from build123d import *

# Parameters (mm, degrees)
SKETCH1_W           = 12
SKETCH1_H           = 18.25
SKETCH2_R           = 3.7145
CUT_EXTRUDE1_DEPTH  = 8.5725
SKETCH3_W           = 73.152
SKETCH3_H           = 124
BOSS_EXTRUDE1_DEPTH = 8
FILLET1_R           = 4
SKETCH6_R           = 13.15
CUT_EXTRUDE2_DEPTH  = 12
SKETCH12_R          = 4.075
CUT_EXTRUDE6_DEPTH  = 2.56
SKETCH12_6_R        = 2.5
CUT_EXTRUDE7_DEPTH  = 8
FILLET2_R           = 0.5
SKETCH13_W          = 73.152
SKETCH13_H          = 13.5
SKETCH13_H_2        = 10
BOSS_EXTRUDE3_DEPTH = 15
FILLET3_R           = 2
SKETCH14_R          = 3.71375
CUT_EXTRUDE8_DEPTH  = 9.5


with BuildPart() as part:
    # Sketch1 → Revolve1 (revolve)
    with BuildSketch(Plane.XY):
        with Locations((14.255, 9.125)):
            Rectangle(SKETCH1_W, SKETCH1_H)
    revolve(axis=Axis((8.255, 0, 0), (1, 0, 0)))

    # Sketch2 → Cut-Extrude1 (cut)
    with BuildSketch(Plane.ZY.offset(-8.255)):
        Circle(SKETCH2_R)
    extrude(amount=-CUT_EXTRUDE1_DEPTH, mode=Mode.SUBTRACT)

    # Sketch6 → Cut-Extrude2 (cut)
    with BuildSketch(Plane.ZY.offset(-8.255)):
        Circle(SKETCH6_R)
    extrude(amount=-CUT_EXTRUDE2_DEPTH, mode=Mode.SUBTRACT)


with BuildPart() as body_2:
    # Sketch3 → Boss-Extrude1 (new body)
    with BuildSketch(Plane(origin=(20.255, 0, 0), x_dir=(0, 0, -1), z_dir=(1, 0, 0))):
        Rectangle(SKETCH3_W, SKETCH3_H)
    extrude(amount=BOSS_EXTRUDE1_DEPTH)

    # Fillet1
    fillet1_edges = [body_2.edges().sort_by_distance(p)[0] for p in [
        (28.255, 0, -36.576),
        (28.255, 0, 36.576),
    ]]
    fillet(fillet1_edges, radius=FILLET1_R)

    # Sketch12 → Cut-Extrude6 (cut)
    with BuildSketch(Plane(origin=(28.255, 0, 0), x_dir=(0, 0, -1), z_dir=(1, 0, 0))):
        Circle(SKETCH12_R)
    extrude(amount=-CUT_EXTRUDE6_DEPTH, mode=Mode.SUBTRACT)

    # Sketch12<6> → Cut-Extrude7 (cut)
    with BuildSketch(Plane(origin=(28.255, 0, 0), x_dir=(0, 0, -1), z_dir=(1, 0, 0))):
        Circle(SKETCH12_6_R)
    extrude(amount=-CUT_EXTRUDE7_DEPTH, mode=Mode.SUBTRACT)

    # Fillet2
    fillet2_edges = [body_2.edges().sort_by_distance(p)[0] for p in [
        (28.255, 0, 4.075),
    ]]
    fillet(fillet2_edges, radius=FILLET2_R)


with BuildPart() as part_1:
    add(part.part)

    # Combine1: union body 2
    add(body_2.part)

    # Sketch13 → Boss-Extrude3 (add)
    with BuildSketch(Plane.ZY.offset(-20.255)):
        with Locations((0, -55.25)):
            Rectangle(SKETCH13_W, SKETCH13_H)
        with Locations((0, 57)):
            Rectangle(SKETCH13_W, SKETCH13_H_2)
    extrude(amount=BOSS_EXTRUDE3_DEPTH)

    # Fillet3
    fillet3_edges = [part_1.edges().sort_by_distance(p)[0] for p in [
        (20.255, -18.25, 0),
        (20.255, 1.75, 36.576),
        (20.255, 1.75, -36.576),
    ]]
    fillet(fillet3_edges, radius=FILLET3_R)

    # Sketch14 → Cut-Extrude8 (cut)
    with BuildSketch(Plane.XZ.offset(62)):
        with Locations((18.52, 12.75)):
            Circle(SKETCH14_R)
        with Locations((18.52, -12.75)):
            Circle(SKETCH14_R)
    extrude(amount=-CUT_EXTRUDE8_DEPTH, mode=Mode.SUBTRACT)


solid = part_1.part
Design review of the part built by this model. Coordinates are the model's own, in mm. A direction names the side the tool comes from. Coordinates: 2 decimals unless noted, no trailing zeros. Loops run counter-clockwise (first coordinate to the right, second up) from the corner with the lowest first, then second, coordinate; pieces in that order, holes last.
Item 1: For faces 4 (the flat face through (20.255, 14, 16)), 5 (the cylindrical face through (22.06, -57.32, -11.63)), 6 (the flat face through (25.695, 2, -2)), list the 3-axis set-ups (+Z, -Z, +X, -X, +Y, -Y) from which the entire face can be reached by the end or side of a thin tool; tool diameter is ignored.
Completed:
face 4: -X
face 5: -Y
face 6: +X
Item 2: Add section C-C (z = 0). Write out the cut boundary in (x, y) (3 decimals).
Completed:
outline: (5.255, -62) - (28.255, -62) - (28.255, -4.575) arc R0.5 ccw to (27.755, -4.075) - (25.695, -4.075) - (25.695, -2.5) - (20.255, -2.5) - (20.255, -13.15) - (8.255, -13.15) - (8.255, -18.25) - (18.255, -18.25) arc R2 cw to (20.255, -20.25) - (20.255, -48.5) - (5.255, -48.5) - close; (5.255, 52) - (20.255, 52) - (20.255, 20.25) arc R2 cw to (18.255, 18.25) - (8.255, 18.25) - (8.255, 13.15) - (20.255, 13.15) - (20.255, 2.5) - (25.695, 2.5) - (25.695, 4.075) - (27.755, 4.075) arc R0.5 ccw to (28.255, 4.575) - (28.255, 62) - (5.255, 62) - close
Item 3: Draft analysis for pull direction Y (two halves, no side actions). For faces 1 (the cylindrical face through (20.52, -57.32, 15.88)), 2 (the flat face through (20.255, -3, 0)), 3 (the flat face through (18, -52.5, -13)), state which applies: pulls with the +Y half, pulls with the -Y half, needs draft (parallel to the pull), parting line crosses it, or undercut.
Completed:
face 1: needs draft
face 2: undercut
face 3: pulls with the -Y half
Item 4: Wall thickness on L1, parallel to Z at x = 18.52, y = -58.5; L2, parallel to Y at x = 15.5, z = 16; L3, parallel to Z at x = 20, y = -53.5: over which ranges is each line inside the solid? List them lowest first.
Completed:
L1: z = -36.58 to -16.46, -9.04 to 9.04, 16.46 to 36.58
L2: y = -62 to -48.5, -8.78 to 8.78, 52 to 62
L3: z = -36.58 to -16.16, -9.34 to 9.34, 16.16 to 36.58
Item 5: Add section D-D (y = 26). Write out the cut boundary in (x, z) (3 decimals).
Completed:
outline: (20.255, -34.576) arc R2 ccw to (22.255, -36.576) - (24.255, -36.576) arc R4 ccw to (28.255, -32.576) - (28.255, 32.576) arc R4 ccw to (24.255, 36.576) - (22.255, 36.576) arc R2 ccw to (20.255, 34.576) - close
Item 6: Add section B-B (y = 0). Write out the cut boundary in (x, z) (3 decimals), and give its area (3 significant figures).
Completed:
outline: (8.255, -18.25) - (18.255, -18.25) arc R2 cw to (20.255, -20.25) - (20.255, -34.576) arc R2 ccw to (22.255, -36.576) - (24.255, -36.576) arc R4 ccw to (28.255, -32.576) - (28.255, -4.575) arc R0.5 ccw to (27.755, -4.075) - (25.695, -4.075) - (25.695, -2.5) - (20.255, -2.5) - (20.255, -13.15) - (8.255, -13.15) - close; (8.255, 13.15) - (20.255, 13.15) - (20.255, 2.5) - (25.695, 2.5) - (25.695, 4.075) - (27.755, 4.075) arc R0.5 ccw to (28.255, 4.575) - (28.255, 32.576) arc R4 ccw to (24.255, 36.576) - (22.255, 36.576) arc R2 ccw to (20.255, 34.576) - (20.255, 20.25) arc R2 cw to (18.255, 18.25) - (8.255, 18.25) - close
area: 653 mm2
Item 7: Clearance check with flat-ended pins moving along their axes: pin 1 (8 mm diameter, centred on y = 0, z = 0, fed in from -X) (3 decimals); pin 2 (4.5 mm diameter, centred on x = 18.52, z = -12.75, fed in from -Y); pin 3 (4 mm diameter, centred on x = 17.5, y = -45.5, fed in from +Z); pin 4 (12 mm diameter, centred on x = 13, y = 3.5, fed in from -Z). State where each tip first meets the part, or that it passes through.
Completed:
pin 1: stops at x = 20.255
pin 2: stops at y = -52.5
pin 3: passes through
pin 4: stops at z = -18.25
Item 8: Add section A-A (x = 9.5). Write out the cut boundary in (y, z), and give its area (3 significant figures).
Completed:
outline: (-62, -36.58) - (-48.5, -36.58) - (-48.5, 36.58) - (-62, 36.58) - close; circle Ø36.5 at (0, 0); (52, -36.58) - (62, -36.58) - (62, 36.58) - (52, 36.58) - close; hole circle Ø26.3 at (0, 0)
area: 2,220 mm2
